For this review, use the dimensioned drawing (mm, ordinates from the lowest corner) and the shaded views. A direction names the side the tool comes from. Coordinates: 2 decimals unless noted, no trailing zeros. Loops run counter-clockwise (first coordinate to the right, second up) from the corner with the lowest first, then second, coordinate; pieces in that order, holes last. Notation, with made-up numbers: (62, -14) -> (86, -14) arc R30 cw to (86, 18) -> close; hole circle Ø10 at (15.25, -25). An arc over 180 degrees is marked (long way). Use one line per item in the form item = value. Start each with the question number.
1. Consider section B-B (y = 20.5). State the section outline as (x, z) points.
2. Consider section A-A (x = 16). State the section outline as (y, z) points, then the cut area to 3 significant figures.
3. Consider section C-C (z = 28.5). State the section outline as (x, y) points, then the cut area to 3 significant figures.
4. Consider section D-D (z = 131). State the section outline as (x, y) points, then the cut area to 3 significant figures.
5. For pin 1 (12 mm diameter, centred on y = 16, z = 100, fed in from +X), flat-tipped, find the tip position at first contact; note if it passes through.
6. Wall thickness on line 1 (Y direction, x = 31.5, z = 100); line 2 (X direction, y = 9.5, z = 134.5): over which ranges is each line inside the solid? List them lowest first. Write a range as from..to.
7. The part is to be moulded in two halves that separate along X. For the marked faces 3, 4 and 5, say which applies: released by +X, released by -X, zero draft, split by the parting line, or undercut.
8. Machinability: for the marked faces 1 and 2, which of the approach directions +Z, -Z, +X, -X, +Y, -Y give a long, thin tool a straight path to every point of the face, cutting with its end or side? Answer none if there is none.
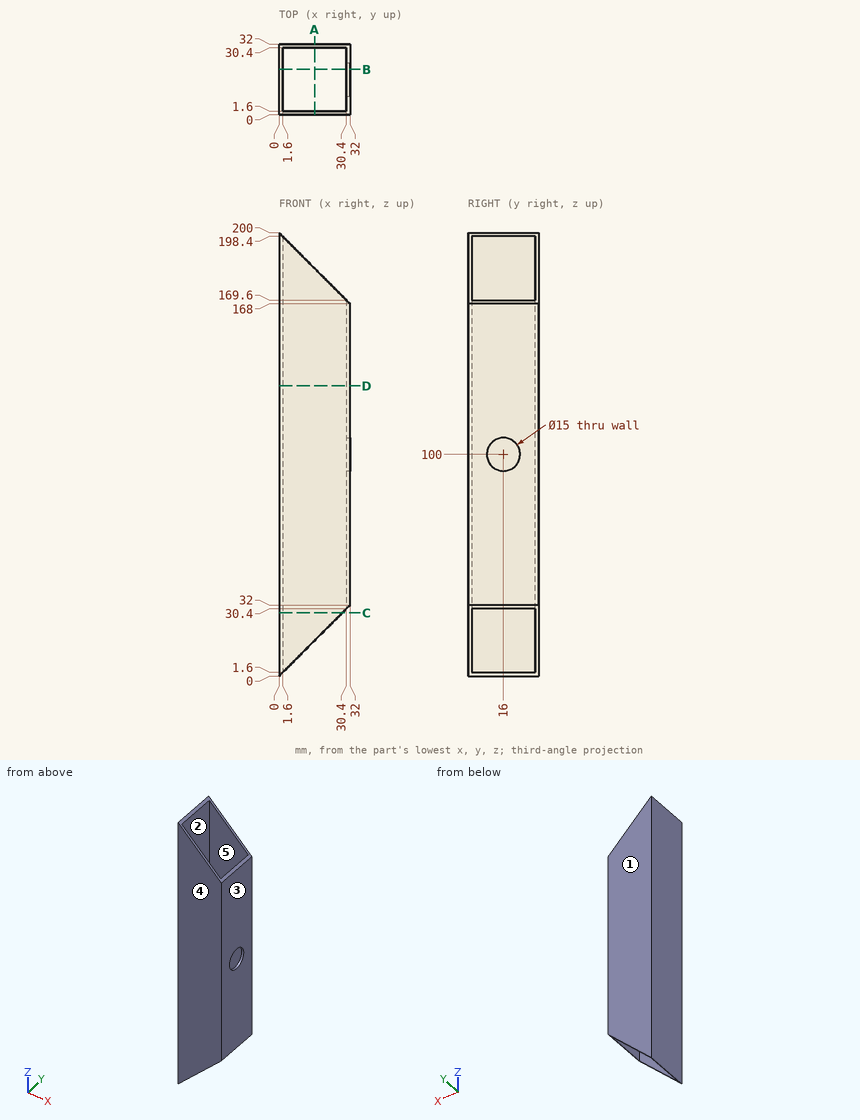
Geometry check:
q1.outline = (0, 0) -> (1.6, 1.6) -> (1.6, 198.4) -> (0, 200) -> close; (30.4, 30.4) -> (32, 32) -> (32, 94) -> (30.4, 94) -> close; (30.4, 106) -> (32, 106) -> (32, 168) -> (30.4, 169.6) -> close
q2.outline = (0, 16) -> (1.6, 16) -> (1.6, 184) -> (0, 184) -> close; (30.4, 16) -> (32, 16) -> (32, 184) -> (30.4, 184) -> close
q2.area = 538 mm²
q3.outline = (0, 0) -> (28.5, 0) -> (28.5, 1.6) -> (1.6, 1.6) -> (1.6, 30.4) -> (28.5, 30.4) -> (28.5, 32) -> (0, 32) -> close
q3.area = 137 mm²
q4.outline = (0, 0) -> (32, 0) -> (32, 32) -> (0, 32) -> close; hole (1.6, 1.6) -> (30.4, 1.6) -> (30.4, 30.4) -> (1.6, 30.4) -> close
q4.area = 195 mm²
q5.pin_1 = 1.6
q6.line_1 = 0..8.5, 23.5..32
q6.line_2 = 0..1.6, 30.4..32
q7.face_3 = released by +X
q7.face_4 = zero draft
q7.face_5 = undercut
q8.face_1 = +Z, -Z, +X, -X, +Y
q8.face_2 = +Z, -Z
